Here's how the part is built. I have some questions about the finished solid (model axes, mm). A direction names the side the tool comes from. Coordinates: 2 decimals unless noted, no trailing zeros. Write each loop counter-clockwise with the first axis right and the second up, starting at its lowest first coordinate (ties: lowest second). Pieces come first, ordered by that corner, then holes.
(1) Imagine slicing it at A-A, the plane y = 19. List the corners of the cut face in (x, z) for me.
(2) Which directions (+Z, -Z, +X, -X, +Y, -Y) give clear straight access to the entire face, cutting with the end or side of a thin tool? Please do faces 4 (the flat face through (123, 50, 0)), 5 (the flat face through (2, 50, -108)), 6 (the flat face through (125, 49, 0)), 7 (the flat face through (-123, 50, -2)), 8 (the flat face through (0, 50, 108)).
(3) Thinking about a two-plate mould opening in X: for faces 1 (the flat face through (-125, 49, -2)), 2 (the flat face through (2, 49, -110)), 3 (the flat face through (-2, 0, -2)), which applies, released by +X, released by -X, zero draft, split by the parting line, or undercut?
(4) Please list where these lines run through material, in increasing order: probe 1 along Z at (x, y) = (-21, 41); probe 2 along X at (y, z) = (89, 57); probe 3 along Y at (x, z) = (100.5, 94.5).
(5) For pin 1 Ø0.6 at (y, z) = (-1.5, -108) entering from -X; pin 2 Ø1 at (y, z) = (-1.5, -108.5) entering from +X, each with a flat end and sliding along its axis, tell me the tip position at first contact or that it passes through.
(6) Imagine slicing it at C-C, the plane x = -15. List the corners of the cut face in (y, z) for me.
(7) Imagine slicing it at B-B, the plane z = -69. List the corners of the cut face in (x, y) for me.
```python
from build123d import *

# Parameters (mm, degrees)
SKETCH_1_W                       = 250
SKETCH_1_H                       = 220
SM_BASE_FLANGE_1_DEPTH           = 2
SM_EDGE_FLANGE_1_STRIP_W         = 9.4732
SM_EDGE_FLANGE_1_STRIP_H         = 2
SM_EDGE_FLANGE_1_STRIP_CUT_DEPTH = 220
SM_EDGE_FLANGE_1_DEPTH           = 220
SM_EDGE_FLANGE_2_STRIP_W         = 9.4732
SM_EDGE_FLANGE_2_STRIP_H         = 2
SM_EDGE_FLANGE_2_STRIP_CUT_DEPTH = 247.2634
SM_EDGE_FLANGE_2_DEPTH           = 247.2634
SM_EDGE_FLANGE_3_STRIP_W         = 9.4732
SM_EDGE_FLANGE_3_STRIP_H         = 2
SM_EDGE_FLANGE_3_STRIP_CUT_DEPTH = 217.2634
SM_EDGE_FLANGE_3_DEPTH           = 217.2634
SM_EDGE_FLANGE_4_STRIP_W         = 9.4732
SM_EDGE_FLANGE_4_STRIP_H         = 2
SM_EDGE_FLANGE_4_STRIP_CUT_DEPTH = 244.5268
SM_EDGE_FLANGE_4_DEPTH           = 244.5268


# Sheet-metal steps are written as plain solids
with BuildPart() as part:
    # Sketch 1 → 基体-法兰1 (new body)
    with BuildSketch(Plane(origin=(0, 0, 0), x_dir=(1, 0, 0), z_dir=(0, 1, 0))):
        Rectangle(SKETCH_1_W, SKETCH_1_H)
    extrude(amount=-SM_BASE_FLANGE_1_DEPTH)

    # 边线-法兰1 strip (across the edge) → 边线-法兰1 strip cut (cut)
    with BuildSketch(Plane(origin=(-125, 0, -110), x_dir=(1, 0, 0), z_dir=(0, 0, 1))):
        with Locations((-2, -1)):
            Rectangle(SM_EDGE_FLANGE_1_STRIP_W, SM_EDGE_FLANGE_1_STRIP_H)
    extrude(amount=SM_EDGE_FLANGE_1_STRIP_CUT_DEPTH, mode=Mode.SUBTRACT)

    # 边线-法兰1 section (across the edge) → 边线-法兰1 (add)
    with BuildSketch(Plane(origin=(-125, 0, -110), x_dir=(1, 0, 0), z_dir=(0, 0, 1))):
        with BuildLine():
            Line((0, 0.7366), (0, 98))
            Line((0, 98), (2, 98))
            Line((2, 98), (2, 0.7366))
            ThreePointArc((2, 0.7366), (2.215745145, 0.215745145), (2.7366, 0))
            Line((2.7366, 0), (2.7366, -2))
            ThreePointArc((2.7366, -2), (0.801531583, -1.198468417), (0, 0.7366))
        make_face()
    extrude(amount=SM_EDGE_FLANGE_1_DEPTH)

    # 边线-法兰2 strip (across the edge) → 边线-法兰2 strip cut (cut)
    with BuildSketch(Plane(origin=(-122.2634, 0, 110), x_dir=(0, 0, -1), z_dir=(1, 0, 0))):
        with Locations((-2, -1)):
            Rectangle(SM_EDGE_FLANGE_2_STRIP_W, SM_EDGE_FLANGE_2_STRIP_H)
    extrude(amount=SM_EDGE_FLANGE_2_STRIP_CUT_DEPTH, mode=Mode.SUBTRACT)

    # 边线-法兰2 section (across the edge) → 边线-法兰2 (add)
    with BuildSketch(Plane(origin=(-122.2634, 0, 110), x_dir=(0, 0, -1), z_dir=(1, 0, 0))):
        with BuildLine():
            Line((0, 0.7366), (0, 98))
            Line((0, 98), (2, 98))
            Line((2, 98), (2, 0.7366))
            ThreePointArc((2, 0.7366), (2.215745145, 0.215745145), (2.7366, 0))
            Line((2.7366, 0), (2.7366, -2))
            ThreePointArc((2.7366, -2), (0.801531583, -1.198468417), (0, 0.7366))
        make_face()
    extrude(amount=SM_EDGE_FLANGE_2_DEPTH)

    # 边线-法兰3 strip (across the edge) → 边线-法兰3 strip cut (cut)
    with BuildSketch(Plane(origin=(125, 0, 107.2634), x_dir=(-1, 0, 0), z_dir=(0, 0, -1))):
        with Locations((-2, -1)):
            Rectangle(SM_EDGE_FLANGE_3_STRIP_W, SM_EDGE_FLANGE_3_STRIP_H)
    extrude(amount=SM_EDGE_FLANGE_3_STRIP_CUT_DEPTH, mode=Mode.SUBTRACT)

    # 边线-法兰3 section (across the edge) → 边线-法兰3 (add)
    with BuildSketch(Plane(origin=(125, 0, 107.2634), x_dir=(-1, 0, 0), z_dir=(0, 0, -1))):
        with BuildLine():
            Line((0, 0.7366), (0, 98))
            Line((0, 98), (2, 98))
            Line((2, 98), (2, 0.7366))
            ThreePointArc((2, 0.7366), (2.215745145, 0.215745145), (2.7366, 0))
            Line((2.7366, 0), (2.7366, -2))
            ThreePointArc((2.7366, -2), (0.801531583, -1.198468417), (0, 0.7366))
        make_face()
    extrude(amount=SM_EDGE_FLANGE_3_DEPTH)

    # 边线-法兰4 strip (across the edge) → 边线-法兰4 strip cut (cut)
    with BuildSketch(Plane(origin=(122.2634, 0, -110), x_dir=(0, 0, 1), z_dir=(-1, 0, 0))):
        with Locations((-2, -1)):
            Rectangle(SM_EDGE_FLANGE_4_STRIP_W, SM_EDGE_FLANGE_4_STRIP_H)
    extrude(amount=SM_EDGE_FLANGE_4_STRIP_CUT_DEPTH, mode=Mode.SUBTRACT)

    # 边线-法兰4 section (across the edge) → 边线-法兰4 (add)
    with BuildSketch(Plane(origin=(122.2634, 0, -110), x_dir=(0, 0, 1), z_dir=(-1, 0, 0))):
        with BuildLine():
            Line((0, 0.7366), (0, 98))
            Line((0, 98), (2, 98))
            Line((2, 98), (2, 0.7366))
            ThreePointArc((2, 0.7366), (2.215745145, 0.215745145), (2.7366, 0))
            Line((2.7366, 0), (2.7366, -2))
            ThreePointArc((2.7366, -2), (0.801531583, -1.198468417), (0, 0.7366))
        make_face()
    extrude(amount=SM_EDGE_FLANGE_4_DEPTH)


solid = part.part
```
Recorded:
1. outline: (-125, -110) - (-123, -110) - (-123, 110) - (-125, 110) - close; (-122.26, -110) - (122.26, -110) - (122.26, -108) - (-122.26, -108) - close; (-122.26, 108) - (125, 108) - (125, 110) - (-122.26, 110) - close; (123, -110) - (125, -110) - (125, 107.26) - (123, 107.26) - close
2. face 4: -Z, +Y
2. face 5: +Y
2. face 6: +Z, -Z, +X, +Y, -Y
2. face 7: +Z, -Z, +Y
2. face 8: +X, +Y
3. face 1: released by -X
3. face 2: zero draft
3. face 3: undercut
4. probe 1: z = -110 to -108, 108 to 110
4. probe 2: x = -125 to -123, 123 to 125
4. probe 3: y = -2 to 0
5. pin 1: stops at x = -124.2
5. pin 2: stops at x = 124.38
6. outline: (-2, -107.26) arc R2.74 ccw to (0.74, -110) - (98, -110) - (98, -108) - (0.74, -108) arc R0.74 cw to (0, -107.26) - (0, 107.26) arc R0.74 cw to (0.74, 108) - (98, 108) - (98, 110) - (0.74, 110) arc R2.74 ccw to (-2, 107.26) - close
7. outline: (-125, 0.74) arc R2.74 ccw to (-122.26, -2) - (122.26, -2) arc R2.74 ccw to (125, 0.74) - (125, 98) - (123, 98) - (123, 0.74) arc R0.74 cw to (122.26, 0) - (-122.26, 0) arc R0.74 cw to (-123, 0.74) - (-123, 98) - (-125, 98) - close
